Geometry: final body of the model. Coordinates: model frame, mm. Face numbers are marked on the shaded views. Give positions to 0.01 mm unless a question says otherwise; leave off trailing zeros. Write each loop counter-clockwise with the first axis right and the second up, starting at its lowest first coordinate (ties: lowest second). Pieces come first, ordered by that corner, then holes.
Q1. Section B-B (z = 0.9). State how many separate pieces and enclosed holes the cut face has, plus the area to 3 significant figures.
Q2. Section A-A (y = 28). Return the cut outline in (x, z).
Q3. Mould query, pull axis Y, two halves, no side actions, for the marked faces 1 and 2. Classes: +Y half, -Y half, draft (parallel to the pull), parting line (faces both ways), or undercut.
Q4. Line query: line 1 (Y direction, x = 9, z = 0.75); line 2 (Y direction, x = 13.5, z = 0.7); line 3 (X direction, y = -4, z = 0.9). Output: solid intervals per line, ascending.
Q5. Pin query (flat end, axial travel): pin 1 Ø1.6 at (y, z) = (35.5, 1.5) entering from +X; pin 2 Ø2 at (y, z) = (-25, 5) entering from +X; pin 3 Ø5 at (x, y) = (0.5, 16.5) entering from +Z. Return the tip coordinate at first contact, or that it passes through.
from build123d import *

# Parameters (mm, degrees)
F0_W      = 50
F0_H      = 90
F1_DEPTH  = 2
F2_R      = 26.5
F3_DEPTH  = 1.5
F4_R      = 26.5
F4_R_2    = 25
F5_DEPTH  = 1
F6_W      = 3
F6_H      = 70
F7_DEPTH  = 3
F8_DEPTH  = 3
F10_DEPTH = 25
F11_W     = 8
F11_H     = 6
F12_DEPTH = 25
F13_R     = 1
F14_R     = 1
F15_R     = 5
F18_SIZE  = 0.25
F19_R     = 26.5
F19_R_2   = 25.25
F19_R_3   = 24.5
F20_DEPTH = 0.5
F21_SIZE  = 0.24999
F22_R     = 26.5
F22_R_2   = 24.74999
F22_R_3   = 24.5
F23_DEPTH = 0.5
F24_SIZE  = 0.2499
F25_R     = 26.5
F25_R_2   = 24.7499
F25_R_3   = 24.5
F26_DEPTH = 0.5
F27_SIZE  = 0.249


# Not quite as in the source:
# - a fillet or chamfer is up to 0.001 mm smaller than in the source, because OpenCascade refuses the exact size


with BuildPart() as f1:
    # F0 (on Top) → F1 (new body)
    with BuildSketch(Plane.XY):
        Rectangle(F0_W, F0_H)
    extrude(amount=F1_DEPTH)

    # F2 (on face) → F3 (join)
    with BuildSketch(Plane.XY.offset(2)):
        Circle(F2_R)
    extrude(amount=F3_DEPTH)

    # F4 (on face) → F5 (join)
    with BuildSketch(Plane.XY.offset(3.5)):
        Circle(F4_R)
        Circle(F4_R_2, mode=Mode.SUBTRACT)
    extrude(amount=F5_DEPTH)

    # F6 (on face) → F7 (join)
    with BuildSketch(Plane(origin=(0, 0, 0), x_dir=(1, 0, 0), z_dir=(0, 0, -1))):
        with Locations((-23.5, 0)):
            Rectangle(F6_W, F6_H)
        with Locations((23.5, 0)):
            Rectangle(F6_W, F6_H)
    extrude(amount=F7_DEPTH)

    # F8 (cut, through all): faces of the model
    f8_faces = [f1.faces().sort_by_distance(p)[0] for p in [
        (-23.5, 0, -3),
        (23.5, 0, -3),
        (-23.5, 0, -3),
        (23.5, 0, -3),
    ]]
    extrude(f8_faces, amount=-F8_DEPTH, mode=Mode.SUBTRACT)

    # F9 (on face) → F10 (cut)
    with BuildSketch(Plane.XY.offset(3.5)):
        with BuildLine():
            Line((-5.6568542495, 0), (-14.8752109279, 9.2183566784))
            ThreePointArc((-14.8752109279, 9.2183566784), (-17.5, 0), (-14.8752109279, -9.2183566784))
            Line((-14.8752109279, -9.2183566784), (-5.6568542495, 0))
        make_face()
        with BuildLine():
            ThreePointArc((-9.2183566784, -14.8752109279), (0, -17.5), (9.2183566784, -14.8752109279))
            Line((9.2183566784, -14.8752109279), (0, -5.6568542495))
            Line((0, -5.6568542495), (-9.2183566784, -14.8752109279))
        make_face()
        with BuildLine():
            ThreePointArc((14.8752109279, -9.2183566784), (16.831015882, -4.7923798244), (17.5, 0))
            ThreePointArc((17.5, 0), (16.831015882, 4.7923798244), (14.8752109279, 9.2183566784))
            Line((14.8752109279, 9.2183566784), (5.6568542495, 0))
            Line((5.6568542495, 0), (14.8752109279, -9.2183566784))
        make_face()
        with BuildLine():
            Line((0, 5.6568542495), (9.2183566784, 14.8752109279))
            ThreePointArc((9.2183566784, 14.8752109279), (0, 17.5), (-9.2183566784, 14.8752109279))
            Line((-9.2183566784, 14.8752109279), (0, 5.6568542495))
        make_face()
    extrude(amount=-F10_DEPTH, mode=Mode.SUBTRACT)

    # F11 (on face) → F12 (cut)
    with BuildSketch(Plane(origin=(0, 0, 0), x_dir=(1, 0, 0), z_dir=(0, 0, -1))):
        with Locations((0, -42)):
            Rectangle(F11_W, F11_H)
        with BuildLine():
            Line((-4, -39), (4, -39))
            Line((4, -39), (19, -39))
            ThreePointArc((19, -39), (19.7071067812, -38.7071067812), (20, -38))
            Line((20, -38), (20, -34))
            ThreePointArc((20, -34), (19.7071067812, -33.2928932188), (19, -33))
            Line((19, -33), (-19, -33))
            ThreePointArc((-19, -33), (-19.7071067812, -33.2928932188), (-20, -34))
            Line((-20, -34), (-20, -38))
            ThreePointArc((-20, -38), (-19.7071067812, -38.7071067812), (-19, -39))
            Line((-19, -39), (-4, -39))
        make_face()
        with Locations((0, 42)):
            Rectangle(F11_W, F11_H)
        with BuildLine():
            ThreePointArc((20, 38), (19.7071067812, 38.7071067812), (19, 39))
            Line((19, 39), (4, 39))
            Line((4, 39), (-4, 39))
            Line((-4, 39), (-19, 39))
            ThreePointArc((-19, 39), (-19.7071067812, 38.7071067812), (-20, 38))
            Line((-20, 38), (-20, 34))
            ThreePointArc((-20, 34), (-19.7071067812, 33.2928932188), (-19, 33))
            Line((-19, 33), (19, 33))
            ThreePointArc((19, 33), (19.7071067812, 33.2928932188), (20, 34))
            Line((20, 34), (20, 38))
        make_face()
    extrude(amount=-F12_DEPTH, mode=Mode.SUBTRACT)

    # F13
    f13_edges = [f1.edges().sort_by_distance(p)[0] for p in [
        (-4, -45, 1),
        (-4, -39, 1),
        (4, -45, 1),
        (4, -39, 1),
    ]]
    fillet(f13_edges, radius=F13_R)

    # F14
    f14_edges = [f1.edges().sort_by_distance(p)[0] for p in [
        (4, 45, 1),
        (4, 39, 1),
        (-4, 45, 1),
        (-4, 39, 1),
    ]]
    fillet(f14_edges, radius=F14_R)

    # F15
    f15_edges = [f1.edges().sort_by_distance(p)[0] for p in [
        (25, -45, 1),
        (25, 45, 1),
        (-25, 45, 1),
        (-25, -45, 1),
    ]]
    fillet(f15_edges, radius=F15_R)


with BuildPart() as f16_1:
    # F16: copy of F1
    add(f1.part.moved(Location((72.1, 0, 0))))


with BuildPart() as f1_1:
    add(f1.part)

    # F18
    f18_edges = [f1_1.edges().sort_by_distance(p)[0] for p in [
        (-25, 0, 4.5),
    ]]
    chamfer(f18_edges, length=F18_SIZE)

    # F19 (on face) → F20 (join)
    with BuildSketch(Plane.XY.offset(4.5)):
        Circle(F19_R)
        Circle(F19_R_2, mode=Mode.SUBTRACT)
        Circle(F19_R_2)
        Circle(F19_R_3, mode=Mode.SUBTRACT)
    extrude(amount=F20_DEPTH)

    # F21 (size 0.25 in the source; OpenCascade refuses exactly that, so slightly less here)
    f21_edges = [f1_1.edges().sort_by_distance(p)[0] for p in [
        (-24.5, 0, 4.5),
        (-24.5, 0, 5),
    ]]
    chamfer(f21_edges, length=F21_SIZE)

    # F22 (on face) → F23 (join)
    with BuildSketch(Plane.XY.offset(5)):
        Circle(F22_R)
        Circle(F22_R_2, mode=Mode.SUBTRACT)
        Circle(F22_R_2)
        Circle(F22_R_3, mode=Mode.SUBTRACT)
    extrude(amount=F23_DEPTH)

    # F24 (size 0.25 in the source; OpenCascade refuses exactly that, so slightly less here)
    f24_edges = [f1_1.edges().sort_by_distance(p)[0] for p in [
        (-24.5, 0, 5),
        (-24.5, 0, 5.5),
    ]]
    chamfer(f24_edges, length=F24_SIZE)

    # F25 (on face) → F26 (join)
    with BuildSketch(Plane.XY.offset(5.5)):
        Circle(F25_R)
        Circle(F25_R_2, mode=Mode.SUBTRACT)
        Circle(F25_R_2)
        Circle(F25_R_3, mode=Mode.SUBTRACT)
    extrude(amount=F26_DEPTH)

    # F27 (size 0.25 in the source; OpenCascade refuses exactly that, so slightly less here)
    f27_edges = [f1_1.edges().sort_by_distance(p)[0] for p in [
        (-24.5, 0, 6),
        (-24.5, 0, 5.5),
    ]]
    chamfer(f27_edges, length=F27_SIZE)


solid = f1_1.part
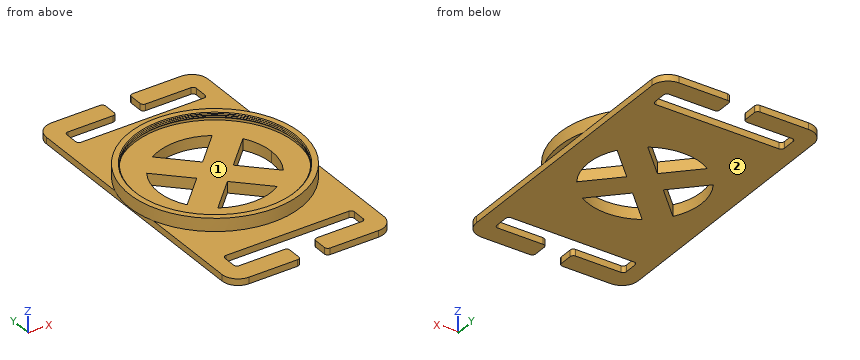
Computed:
1. separate pieces: 1
1. enclosed holes: 4
1. area: 3,430 mm2
2. outline: (-25, 0) - (25, 0) - (25, 2) - (-25, 2) - close
3. face 1: undercut
3. face 2: draft
4. line 1: y = -45 to -39, -33 to -15.01, -14.66 to -3.34, 3.34 to 14.66, 15.01 to 33, 39 to 45
4. line 2: y = -45 to -39, -33 to -7.84, 7.84 to 33, 39 to 45
4. line 3: x = -25 to -17.04, -9.66 to 9.66, 17.04 to 25
5. pin 1: stops at x = 25
5. pin 2: stops at x = 11.24
5. pin 3: stops at z = 3.5
